Geometry: final body of the model. Coordinates: model frame, mm. Coordinates: 2 decimals unless noted, no trailing zeros. Write each loop counter-clockwise with the first axis right and the second up, starting at its lowest first coordinate (ties: lowest second). Pieces come first, ordered by that corner, then holes.
from build123d import *

# Parameters (mm, degrees)
SKETCH1_W                                          = 69.85
SKETCH1_H                                          = 44.45
BOSS_EXTRUDE1_DEPTH                                = 9.525
CSK_FOR_10_FLAT_HEAD_MACHINE_SCREW_100_D           = 5.1054
CSK_FOR_10_FLAT_HEAD_MACHINE_SCREW_100_CSINK_D     = 9.779
CSK_FOR_10_FLAT_HEAD_MACHINE_SCREW_100_CSINK_ANGLE = 82
F_10_0_2_DIAMETER_HOLE1_D                          = 5.08
FILLET4_R                                          = 6.35


with BuildPart() as part:
    # Sketch1 → Boss-Extrude1 (new body)
    with BuildSketch(Plane(origin=(0, 0, 0), x_dir=(1, 0, 0), z_dir=(0, 1, 0))):
        Rectangle(SKETCH1_W, SKETCH1_H)
    extrude(amount=BOSS_EXTRUDE1_DEPTH)

    # CSK for #10 Flat Head Machine Screw (100)1 (through all)
    with Locations(Plane(origin=(0, 0, 0), x_dir=(-1, 0, 0), z_dir=(0, -1, 0))):
        with Locations((0, 11.1125), (0, -11.1125)):
            CounterSinkHole(CSK_FOR_10_FLAT_HEAD_MACHINE_SCREW_100_D / 2, CSK_FOR_10_FLAT_HEAD_MACHINE_SCREW_100_CSINK_D / 2, counter_sink_angle=CSK_FOR_10_FLAT_HEAD_MACHINE_SCREW_100_CSINK_ANGLE)

    # #10 (0.2) Diameter Hole1 (through all)
    with Locations(Plane(origin=(0, 0, 0), x_dir=(-1, 0, 0), z_dir=(0, -1, 0))):
        with Locations((-25.4, 0)):
            f_10_0_2_diameter_hole1 = Hole(F_10_0_2_DIAMETER_HOLE1_D / 2)

    # Mirror1: #10 (0.2) Diameter Hole1 across plane
    add(f_10_0_2_diameter_hole1.mirror(Plane(origin=(0, 0, 0), x_dir=(0, 0, 1), z_dir=(1, 0, 0))), mode=Mode.SUBTRACT)

    # Fillet4
    fillet4_edges = [part.edges().sort_by_distance(p)[0] for p in [
        (34.925, 4.7625, 22.225),
        (-34.925, 4.7625, 22.225),
        (-34.925, 4.7625, -22.225),
        (34.925, 4.7625, -22.225),
    ]]
    fillet(fillet4_edges, radius=FILLET4_R)


solid = part.part
Item 1: Material intervals for probe 1 along Z at (x, y) = (0, 5.5) (3 decimals); probe 2 along Z at (x, y) = (25.4, 5.75) (3 decimals); probe 3 along X at (y, z) = (8.5, 1) (3 decimals), sorted ascending.
Derived:
probe 1: z = -22.225 to -13.665, -8.56 to 8.56, 13.665 to 22.225
probe 2: z = -22.225 to -2.54, 2.54 to 22.225
probe 3: x = -34.925 to -27.735, -23.065 to 23.065, 27.735 to 34.925
Item 2: Section C-C, the plane x = 0. Output: boundary loops of the cut face in (y, z) (3 decimals).
Derived:
outline: (0, -22.225) - (9.525, -22.225) - (9.525, -13.665) - (2.688, -13.665) - (0, -16.002) - close; (0, -6.223) - (2.688, -8.56) - (9.525, -8.56) - (9.525, 8.56) - (2.688, 8.56) - (0, 6.223) - close; (0, 16.002) - (2.688, 13.665) - (9.525, 13.665) - (9.525, 22.225) - (0, 22.225) - close
Item 3: Pin query (flat end, axial travel): pin 1 (6 mm diameter, centred on x = 0, z = 11.11, fed in from +Y) (3 decimals); pin 2 (8 mm diameter, centred on x = 0, z = -11.11, fed in from -Y). Return the tip coordinate at first contact, or that it passes through.
Derived:
pin 1: stops at y = 9.525
pin 2: stops at y = 1.02
Item 4: Section B-B, the plane x = -25.4. Output: boundary loops of the cut face in (y, z) (3 decimals), plus the area to 3 significant figures.
Derived:
outline: (0, -22.225) - (9.525, -22.225) - (9.525, -2.54) - (0, -2.54) - close; (0, 2.54) - (9.525, 2.54) - (9.525, 22.225) - (0, 22.225) - close
area: 375 mm2
Item 5: Pull-direction query (Z, two-part tool) for faces 1 (the flat face through (-34.925, 5, 0)), 2 (the flat face through (0, 5, 22.225)), 3 (the flat face through (0, 5, -22.225)), 4 (the cylindrical face through (-27.823, 4.829, -0.763)); classes: released by +Z, released by -Z, zero draft, split by the parting line, or undercut.
Derived:
face 1: zero draft
face 2: released by +Z
face 3: released by -Z
face 4: undercut
Item 6: Section D-D, the plane y = 6.75. State how many separate pieces and enclosed holes the cut face has, plus the area to 3 significant figures.
Derived:
separate pieces: 1
enclosed holes: 4
area: 2,990 mm2
Item 7: Section A-A, the plane z = 0. Output: boundary loops of the cut face in (x, y) (3 decimals), plus the area to 3 significant figures.
Derived:
outline: (-34.925, 0) - (-27.94, 0) - (-27.94, 9.525) - (-34.925, 9.525) - close; (-22.86, 0) - (22.86, 0) - (22.86, 9.525) - (-22.86, 9.525) - close; (27.94, 0) - (34.925, 0) - (34.925, 9.525) - (27.94, 9.525) - close
area: 569 mm2
